```python
from build123d import *

# Parameters (mm, degrees)
CHANFREIN1_SIZE = 0.75


with BuildPart() as part:
    # Esquisse1 → Base-Révolution (revolve)
    with BuildSketch(Plane.XY, mode=Mode.PRIVATE) as base_r_volution_sk:
        with BuildLine():
            Line((0, 6), (10, 6))
            Line((10, 6), (10, 5))
            Line((10, 5), (12, 5))
            Line((12, 5), (12, 6))
            Line((12, 6), (14, 6))
            Line((14, 6), (14, 3))
            Line((14, 3), (36, 3))
            Line((36, 3), (36, 0))
            Line((36, 0), (-1.66190379, 0))
            ThreePointArc((-1.66190379, 0), (-1.238750773, 3.11295375), (0, 6))
        make_face()
    revolve(base_r_volution_sk.sketch.rotate(Axis((-3, 0, 0), (1, 0, 0)), 180), axis=Axis((-3, 0, 0), (1, 0, 0)))

    # Chanfrein1
    chanfrein1_edges = [part.edges().sort_by_distance(p)[0] for p in [
        (36, 3, 0),
    ]]
    chamfer(chanfrein1_edges, length=CHANFREIN1_SIZE)


solid = part.part
```
Part model, mm, in its own coordinate system. A direction names the side the tool comes from. Coordinates: 2 decimals unless noted, no trailing zeros. Write each loop counter-clockwise with the first axis right and the second up, starting at its lowest first coordinate (ties: lowest second). Pieces come first, ordered by that corner, then holes.
Item 1: Mould opens along X. For faces 4 (the face through (13.014, -5.723, -1.802)), 5 (the face through (10, 4, -4)), 6 (the face through (14, 3, 1)) say: released by +X, released by -X, zero draft, split by the parting line, or undercut.
Item 2: Pin check, flat tips, straight feed: pin 1 (1 mm diameter, centred on y = 1.5, z = -4.5, fed in from -X); pin 2 (2 mm diameter, centred on y = 2, z = 2, fed in from -X); pin 3 (5 mm diameter, centred on y = 1.5, z = 3.5, fed in from -X); pin 4 (3.5 mm diameter, centred on y = 1, z = 0.5, fed in from -X). Stop position of each tip, or through.
Item 3: Slice it at D-D (z = -3.5). Write the cut outline in (x, y).
Item 4: Slice it at C-C (x = 9). Write the cut outline in (y, z), and give its area (3 significant figures).
Item 5: Probe line 1 (X direction, y = 1.5, z = 5); line 2 (X direction, y = -4.75, z = -2); line 3 (X direction, y = 2.25, z = 2.75). List the from-to ranges inside material, lowest first.
Item 6: Which spindle directions (+Z, -Z, +X, -X, +Y, -Y) get a long thin tool onto all of the face, cutting with end or side? Do faces 1 (the face through (12, -4, -4)), 2 (the face through (24.77, -2.86, -0.9)), 3 (the face through (36, 0, 0)). Say none if no direction does.
Item 7: Slice it at A-A (z = 0). Write the cut outline in (x, y).
Results found:
1. face 4: zero draft
1. face 5: undercut
1. face 6: released by +X
2. pin 1: stops at x = -0.86
2. pin 2: stops at x = -1.52
2. pin 3: stops at x = -1.59
2. pin 4: stops at x = -1.66
3. outline: (0, -4.87) - (10, -4.87) - (10, -3.57) - (12, -3.57) - (12, -4.87) - (14, -4.87) - (14, 4.87) - (12, 4.87) - (12, 3.57) - (10, 3.57) - (10, 4.87) - (0, 4.87) arc R11.12 ccw to start
4. outline: circle Ø12 at (0, 0)
4. area: 113 mm2
5. line 1: x = -0.43 to 10, 12 to 14
5. line 2: x = -0.46 to 10, 12 to 14
5. line 3: x = -1.11 to 14
6. face 1: none
6. face 2: +X
6. face 3: +Z, -Z, +X, +Y, -Y
7. outline: (0, -6) - (10, -6) - (10, -5) - (12, -5) - (12, -6) - (14, -6) - (14, -3) - (35.25, -3) - (36, -2.25) - (36, 2.25) - (35.25, 3) - (14, 3) - (14, 6) - (12, 6) - (12, 5) - (10, 5) - (10, 6) - (0, 6) arc R11.66 ccw to start
